```python
from build123d import *

# Parameters (mm, degrees)
F0_W     = 51
F0_H     = 26
F0_W_2   = 46.5
F0_H_2   = 21.5
F1_DEPTH = 2
F2_DEPTH = 4
F3_R     = 1.5
F4_R     = 1.5


with BuildPart() as f1:
    # F0 (on Top) → F1 (new body)
    with BuildSketch(Plane.XY):
        Rectangle(F0_W, F0_H)
        Rectangle(F0_W_2, F0_H_2, mode=Mode.SUBTRACT)
    extrude(amount=F1_DEPTH)

    # F0 (on Top) → F2 (join)
    with BuildSketch(Plane.XY):
        Rectangle(F0_W_2, F0_H_2)
    extrude(amount=F2_DEPTH)

    # F3
    f3_edges = [f1.edges().sort_by_distance(p)[0] for p in [
        (25.5, 13, 1),
        (-25.5, 13, 1),
        (-25.5, -13, 1),
        (25.5, -13, 1),
        (25.5, 0, 0),
        (0, -13, 0),
        (-25.5, 0, 0),
        (0, 13, 0),
    ]]
    fillet(f3_edges, radius=F3_R)

    # F4
    f4_edges = [f1.edges().sort_by_distance(p)[0] for p in [
        (-23.25, -10.75, 3),
        (-23.25, 10.75, 3),
        (23.25, 10.75, 3),
        (23.25, -10.75, 3),
        (23.25, 0, 4),
        (0, -10.75, 4),
        (-23.25, 0, 4),
        (0, 10.75, 4),
    ]]
    fillet(f4_edges, radius=F4_R)


solid = f1.part
```
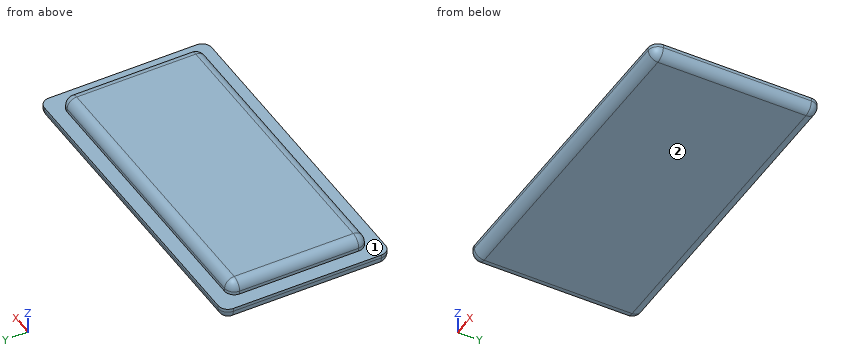
Geometry: final body of the model. Coordinates: model frame, mm. Face numbers are marked on the shaded views. A direction names the side the tool comes from. Give positions to 0.01 mm unless a question says otherwise; leave off trailing zeros. Order: outer loops, then holes, each group sorted by start corner. A loop starts at its lowest first (then second) coordinate and runs counter-clockwise, first axis right, second up. Notation, with made-up numbers: M 16,81 L 73,81 A19 ccw 73,103 Z; hole C 0.25,51.5 d6. An arc over 180 degrees is marked long. Answer as CSV lines item,"result". Start each with the question number.
1) Line query: line 1 (Y direction, x = -8, z = 1.4); line 2 (Y direction, x = 3, z = 2.5); line 3 (X direction, y = 3.75, z = 2.55). Output: solid intervals per line, ascending. Write a range as from..to.
2) Set-up query: the marked faces 1 and 2. Return all of +Z, -Z, +X, -X, +Y, -Y with unobstructed straight access to the full face (end or side cutting, diameter ignored); none if empty.
3) Cut plane A-A (x = -11.5). Output: boundary loops of the cut face in (y, z).
4) Cut plane B-B (y = 3.25). Output: boundary loops of the cut face in (x, z).
Findings below:
1,line 1,"y = -13..13"
1,line 2,"y = -10.75..10.75"
1,line 3,"x = -23.25..23.25"
2,face 1,"+Z"
2,face 2,"-Z, +X, -X, +Y, -Y"
3,outline,"M -13,1.5 A1.5 ccw -11.5,0 L 11.5,0 A1.5 ccw 13,1.5 L 13,2 L 10.75,2 L 10.75,2.5 A1.5 ccw 9.25,4 L -9.25,4 A1.5 ccw -10.75,2.5 L -10.75,2 L -13,2 Z"
4,outline,"M -25.5,1.5 A1.5 ccw -24,0 L 24,0 A1.5 ccw 25.5,1.5 L 25.5,2 L 23.25,2 L 23.25,2.5 A1.5 ccw 21.75,4 L -21.75,4 A1.5 ccw -23.25,2.5 L -23.25,2 L -25.5,2 Z"
